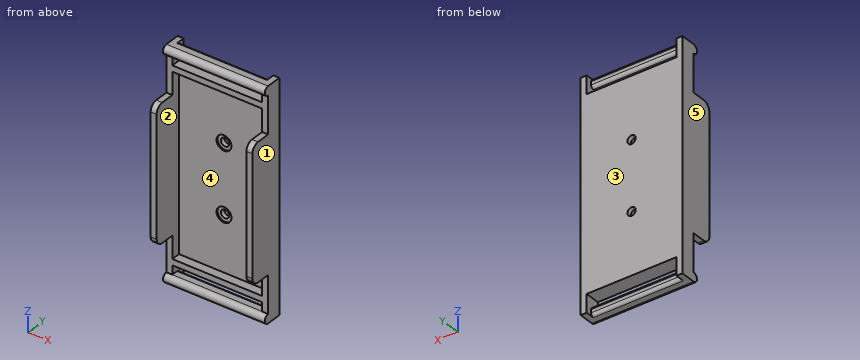
Autodesk Inventor part; units mm, degrees
ref_plane "YZ Plane" through (0, 0, 0) normal (1, 0, 0) x (0, 1, 0)
ref_plane "XZ Plane" through (0, 0, 0) normal (0, 1, 0) x (-1, 0, 0)
ref_plane "XY Plane" through (0, 0, 0) normal (0, 0, 1) x (1, 0, 0)
sketch "Sketch1" plane through (0, 0, 0) normal (0, 1, 0) x (-1, 0, 0)
  line L0 (15, 30) -> (-15, 30)
  line L1 (-15, 30) -> (-15, -30)
  line L2 (-15, -30) -> (15, -30)
  line L3 (15, -30) -> (15, 30)
  line L4 (0, 11.5) -> (-15, 11.5)
  line L5 (-15, 11.5) -> (-15, -11.5)
  line L6 (-15, -11.5) -> (0, -11.5)
  line L7 (0, -11.5) -> (0, 11.5)
  point P0 (0, 0)
  dimension "d0" = 30
  dimension "d1" = 60
  dimension "d2" = 30
  dimension "d3" = 15
  dimension "d4" = 23
  dimension "d5" = 18.5
extrude "Extrusion1" add sketch "Sketch1" along normal blind 2
hole "Hole1" at (0, 0, -11.5) at (0, 0, 11.5) direction (0, 1, 0) diameter 2.8 end through all counterbore diameter 5 counterbore depth 0.5
sketch "Sketch2" plane through (0, 0, 0) normal (0, -1, 0) x (1, 0, 0)
  line L0 (17, 32) -> (-17, 32)
  line L1 (-17, 32) -> (-17, -32)
  line L2 (-17, -32) -> (17, -32)
  line L3 (17, -32) -> (17, 32)
  line L4 (15, 30) -> (15, -30)
  line L5 (-15, -30) -> (-15, 30)
  line L6 (15, 30) -> (-15, 30)
  line L7 (-15, 30) -> (-15, -30)
  line L8 (-15, -30) -> (15, -30)
  line L9 (15, -30) -> (15, 30)
  point P0 (0, 0)
  point P1 (-15, 30)
  dimension "d15" = 34
  dimension "d16" = 64
  dimension "d17" = 32
  dimension "d18" = 17
extrude "Extrusion2" add sketch "Sketch2" along normal blind 3 and the other way blind 2
sketch "Sketch3" plane through (-17, -3, -32) normal (-1, 0, 0) x (0, 0, 1)
  line L0 (2, 0) -> (62, 0)
  line L1 (54.5, 0) -> (9.5, 0)
  line L2 (9.5, 0) -> (9.5, -7)
  line L3 (9.5, -7) -> (54.5, -7)
  line L4 (54.5, -7) -> (54.5, 0)
  line L5 (2, 3) -> (62, 3)
  line L6 (64, 0) -> (64, 5)
  circle A0 centre (52, -4.5) radius 2.5
  circle A1 centre (12, -4.5) radius 2.5
  point P0 (32, 3)
  point P1 (52, -7)
  point P2 (54.5, -4.5)
  point P3 (9.5, 0)
  point P4 (9.5, -4.5)
  point P5 (12, -7)
  dimension "d23" = 10
  dimension "d24" = 45
  dimension "d25" = 9.5
  dimension "d26" = 5
  dimension "d27" = 5
  dimension "d28" = 2.5
  dimension "d29" = 2.5
extrude "Extrusion3" add sketch "Sketch3" against normal up to surface (2 mm away) contours L0 L4 A0 L3 A1 L2 | A1 | A0
mirror "Mirror1" about plane through (0, 0, 0) normal (1, 0, 0) of "Extrusion3"
sketch "Sketch6" plane through (0, -3, 0) normal (0, -1, 0) x (1, 0, 0)
  line L0 (15, 30) -> (-15, 30)
  line L1 (-15, 30) -> (-15, 35)
  line L2 (-15, 35) -> (15, 35)
  line L3 (15, 35) -> (15, 30)
  line L4 (17, 32) -> (-17, 32)
  line L5 (17, 32) -> (-17, 32)
  line L6 (-17, 32) -> (-17, 38)
  line L7 (-17, 38) -> (17, 38)
  line L8 (17, 38) -> (17, 32)
  point P0 (0, 0)
  point P1 (15, 32)
  point P2 (-15, 32)
  dimension "d34" = 3
  dimension "d35" = 6
extrude "Extrusion4" add sketch "Sketch6" against normal up to surface (5 mm away) contours L3 L2 L1 L4 L6 L7 L8
sketch "Sketch7" plane through (0, 2, 0) normal (0, 1, 0) x (1, 0, 0)
  line L0 (-15, -35) -> (15, -35)
  line L1 (17, -38) -> (-17, -38)
  line L2 (15, -35) -> (-14.9996, -35)
  line L3 (-14.9996, -35) -> (-14.9996, -38)
  line L4 (-14.9996, -38) -> (15, -38)
  line L5 (15, -38) -> (15, -35)
  point P0 (0, 0)
extrude "Extrusion5" cut sketch "Sketch7" against normal blind 2
sketch "Sketch8" plane through (-17, -3, -32) normal (-1, 0, 0) x (0, 0, 1)
  line L0 (70, 0) -> (54.5, 0)
  circle A0 centre (68.5, 0) radius 1.5
  point P0 (32, 3)
  point P1 (67, 0)
  dimension "d41" = 3
extrude "Extrusion6" add sketch "Sketch8" against normal up to surface (34 mm away) contours A0 L0 picked at (68.5603, -0.4964)
mirror "Mirror2" about plane through (0, 0, 0) normal (0, 0, 1) of "Extrusion4", "Extrusion5", "Extrusion6"
fillet "Fillet2" radius 1 4 edges at (0.0002, 0, -38) (0.0002, 0, -35) (0.0002, 0, 38) (0.0002, 0, 35)
equation "\"d5\" = -0.5 * d4 + 0.5 * d1"
properties part number "Battery_holder_2"
Read the model definition and answer for the solid it produces. Units are mm, in the model's axes. Face numbers are marked on the shaded views. A direction names the side the tool comes from. Coordinates: 2 decimals unless noted, no trailing zeros. Loops run counter-clockwise (first coordinate to the right, second up) from the corner with the lowest first, then second, coordinate; pieces in that order, holes last. Notation, with made-up numbers: (58.25, -24) - (103.25, -24) arc R11 ccw to (103.25, -20) - close; hole circle Ø8 at (61.25, 36.5). An arc over 180 degrees is marked (long way). Answer in a Markdown table with one row per item.
Q1. Find section A-A on x = -10. Write down the section's boundary in (y, z).
Here are the results:
| item | result |
|---|---|
| outline | (-3, -38) - (-1, -38) arc R1 ccw to (0, -37) - (0, -36) arc R1 ccw to (-1, -35) - (-3, -35) arc R1.5 ccw to start; (-3, -32) - (2, -32) - (2, 32) - (-3, 32) - (-3, 30) - (0, 30) - (0, -30) - (-3, -30) - close; (-3, 35) - (-1, 35) arc R1 ccw to (0, 36) - (0, 37) arc R1 ccw to (-1, 38) - (-3, 38) arc R1.5 ccw to start |
Q2. Straight lines are drawn through the part: line 1 along Z through (x, y) = (0, 0.8); line 2 along Z through (x, y) = (0, 0.4); line 3 along Z through (x, y) = (9.5, -2.75). For each, find the intervals that lie inside material, in ascending order. Write a range as [from, to].
Here are the results:
| item | result |
|---|---|
| line 1 | z = [-32, -12.9], [-10.1, 10.1], [12.9, 32] |
| line 2 | z = [-32, -14], [-9, 9], [14, 32] |
| line 3 | z = [-38, -35], [-32, -30], [30, 32], [35, 38] |
Q3. Find section B-B on z = 11.5. Write down the section's boundary in (x, y).
Here are the results:
| item | result |
|---|---|
| outline | (-17, -10) - (-15, -10) - (-15, 0) - (-2.5, 0) - (-2.5, 0.5) - (-1.4, 0.5) - (-1.4, 2) - (-17, 2) - close; (1.4, 0.5) - (2.5, 0.5) - (2.5, 0) - (15, 0) - (15, -10) - (17, -10) - (17, 2) - (1.4, 2) - close |
Q4. For the marked faces 1 and 2, determine the directions among +Z, -Z, +X, -X, +Y, -Y from which every point of the face is accessible in a straight line to the end or side of a thin tool.
Here are the results:
| item | result |
|---|---|
| face 1 | +Z, -Z, +X, +Y, -Y |
| face 2 | -Y |
Q5. The mould has two halves that part along X. Classify the marked faces 3, 4 and 5: pulls with the +X half, pulls with the -X half, needs draft (parallel to the pull), parting line crosses it, or undercut.
Here are the results:
| item | result |
|---|---|
| face 3 | needs draft |
| face 4 | undercut |
| face 5 | pulls with the -X half |
Q6. Find section D-D on z = -6.5. Write down the section's boundary in (x, y), plus the area to 3 significant figures.
Here are the results:
| item | result |
|---|---|
| outline | (-17, -10) - (-15, -10) - (-15, 0) - (15, 0) - (15, -10) - (17, -10) - (17, 2) - (-17, 2) - close |
| area | 108 mm^2 |
Q7. Given P1, Ø2, axis at x = -15.5, y = -5, coming from the -Z side; P2, Ø0.6, axis at x = 16, y = -5, coming from the +Z side; P3, Ø0.5, axis at x = -1, z = -36.5, coming from the +Y side, each flat-ended and moving along its own axis, determine where each tip first touches the part or whether it passes through.
Here are the results:
| item | result |
|---|---|
| P1 | stops at z = -37.62 |
| P2 | stops at z = 22.5 |
| P3 | stops at y = 0 |
Q8. Find section C-C on y = -9.25. Write down the section's boundary in (x, z), plus the area to 3 significant figures.
Here are the results:
| item | result |
|---|---|
| outline | (-17, -21.79) - (-15, -21.79) - (-15, 21.79) - (-17, 21.79) - close; (15, -21.79) - (17, -21.79) - (17, 21.79) - (15, 21.79) - close |
| area | 174 mm^2 |
